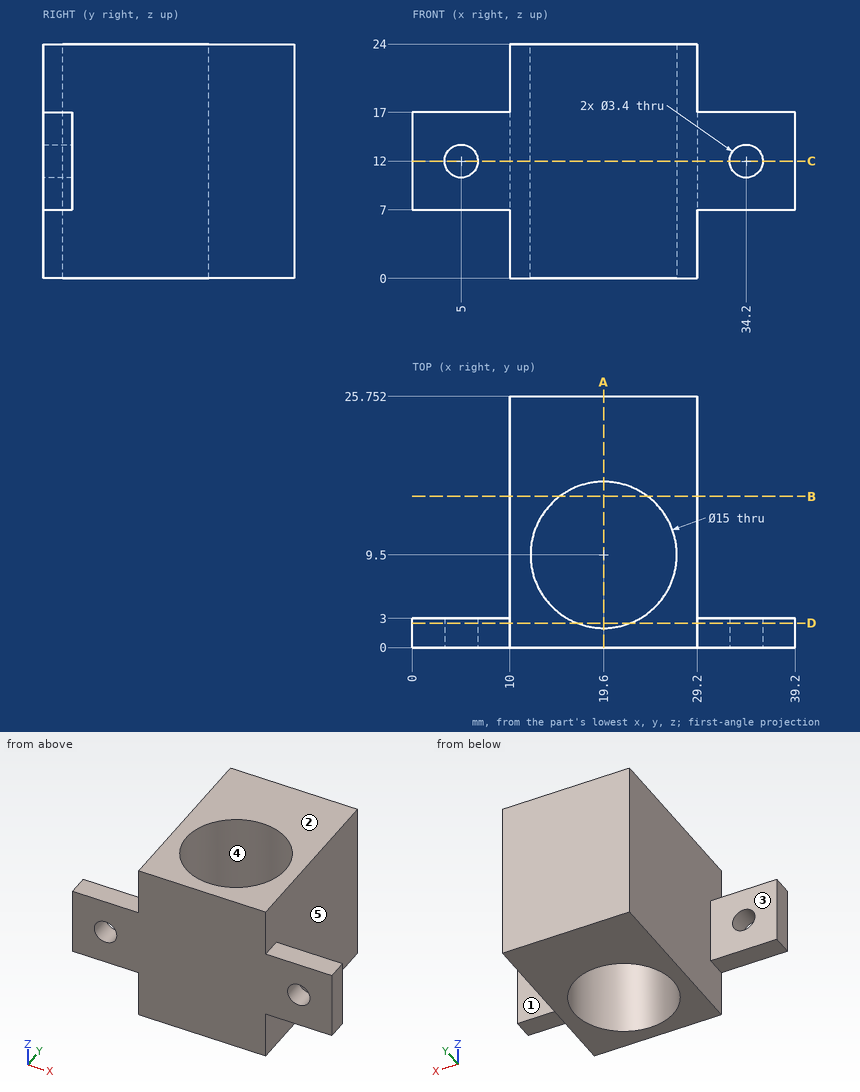
Geometry: see drawing. Coordinates: mm, zero at the bounding-box minimum. A direction names the side the tool comes from. Give positions to 0.01 mm unless a question says otherwise; leave off trailing zeros. Loops run counter-clockwise (first coordinate to the right, second up) from the corner with the lowest first, then second, coordinate; pieces in that order, holes last. Notation, with made-up numbers: (35.25, -13.5) -> (50.25, -13.5) arc R28 cw to (50.25, 21.5) -> close; hole circle Ø10 at (-0.75, 74.25). An arc over 180 degrees is marked (long way). Put each result on its own line as item: value.
1. Set-up query: the marked faces 1 and 2. Return all of +Z, -Z, +X, -X, +Y, -Y with unobstructed straight access to the full face (end or side cutting, diameter ignored); none if empty.
Taken from the geometry:
face 1: +Z, -Z, +X, +Y
face 2: +Z, +X, -X, +Y, -Y
2. Ray query, line 1 along X through (y, z) = (1.4, 12); line 2 along Y through (x, z) = (19.6, 5); line 3 along Y through (x, z) = (8, 13.75). Return the intervals inside material, ascending. Write a range as [from, to].
Taken from the geometry:
line 1: x = [0, 3.3], [6.7, 32.5], [35.9, 39.2]
line 2: y = [0, 2], [17, 25.75]
line 3: y = [0, 3]
3. Pull-direction query (Y, two-part tool) for the marked faces 3, 4 and 5; classes: released by +Y, released by -Y, zero draft, split by the parting line, or undercut.
Taken from the geometry:
face 3: released by +Y
face 4: undercut
face 5: zero draft
4. Cut plane C-C (z = 12). Return the cut outline in (x, y), plus the area to 3 significant figures.
Taken from the geometry:
outline: (0, 0) -> (3.3, 0) -> (3.3, 3) -> (0, 3) -> close; (6.7, 0) -> (32.5, 0) -> (32.5, 3) -> (29.2, 3) -> (29.2, 25.75) -> (10, 25.75) -> (10, 3) -> (6.7, 3) -> close; (35.9, 0) -> (39.2, 0) -> (39.2, 3) -> (35.9, 3) -> close; hole circle Ø15 at (19.6, 9.5)
area: 357 mm2
5. Cut plane A-A (x = 19.6). Return the cut outline in (y, z), plus the area to 3 significant figures.
Taken from the geometry:
outline: (0, 0) -> (2, 0) -> (2, 24) -> (0, 24) -> close; (17, 0) -> (25.75, 0) -> (25.75, 24) -> (17, 24) -> close
area: 258 mm2
6. Cut plane D-D (y = 2.5). Return the cut outline in (x, z), plus the area to 3 significant figures.
Taken from the geometry:
outline: (0, 7) -> (10, 7) -> (10, 0) -> (16.91, 0) -> (16.91, 24) -> (10, 24) -> (10, 17) -> (0, 17) -> close; (22.29, 0) -> (29.2, 0) -> (29.2, 7) -> (39.2, 7) -> (39.2, 17) -> (29.2, 17) -> (29.2, 24) -> (22.29, 24) -> close; hole circle Ø3.4 at (5, 12); hole circle Ø3.4 at (34.2, 12)
area: 513 mm2
7. Cut plane B-B (y = 15.5). Return the cut outline in (x, z).
Taken from the geometry:
outline: (10, 0) -> (15.1, 0) -> (15.1, 24) -> (10, 24) -> close; (24.1, 0) -> (29.2, 0) -> (29.2, 24) -> (24.1, 24) -> close
8. Pin query (flat end, axial travel): P1, Ø2.5, axis at x = 5, y = 1.5, coming from the +Z side; P2, Ø12, axis at y = 11, z = 11, coming from the -X side; P3, Ø12, axis at y = 18, z = 15.5, coming from the +X side. Return the tip coordinate at first contact, or that it passes through.
Taken from the geometry:
P1: stops at z = 17
P2: stops at x = 10
P3: stops at x = 29.2
